Part model, mm, in its own coordinate system. Coordinates: 2 decimals unless noted, no trailing zeros. Order: outer loops, then holes, each group sorted by start corner. A loop starts at its lowest first (then second) coordinate and runs counter-clockwise, first axis right, second up.
from build123d import *

# Parameters (mm, degrees)
BOSS_EXTRUDE1_DEPTH = 129
FILLET1_R           = 0.2
FILLET1_R_2         = 0.3
FILLET1_R_3         = 1
FILLET1_R_4         = 0.5
CHAMFER1_SIZE       = 0.8
CHAMFER1_SIZE2      = 0.601769912


with BuildPart() as part:
    # Sketch1 → Boss-Extrude1 (new body)
    with BuildSketch(Plane.XY):
        Polygon((1.5, 20.5), (1.5, 5.5), (2.375, 5.5), (4.125, 2.75), (5.875, 5.5), (8.5, 5.5), (8.5, 20.5), (9.25, 20.5), (10, 17.8), (10, 0), (8.5, 0), (6.75, 4), (3.25, 0), (1.5, 4), (0, 4), (0, 17.8), (0.75, 20.5), align=None)
    extrude(amount=BOSS_EXTRUDE1_DEPTH)

    # Fillet1
    # the kernel refuses this fillet: 1, 0.5, 0.3, 0.2 mm, written as the material it adds along each edge
    with BuildSketch(Plane(origin=(6.75, 4, 0), x_dir=(0.40081883401970875, -0.9161573349021888, 0), z_dir=(0, 0, 1))) as fillet1_piece_1:
        with BuildLine():
            CenterArc((FILLET1_R * 1.57528283018, -FILLET1_R), FILLET1_R, 90, 115.184697104)
            Line((FILLET1_R * 0.670342090327, -FILLET1_R * 1.42553760981), (0, 0))
            Line((0, 0), (FILLET1_R * 1.57528283018, 0))
        make_face()
    extrude(amount=129)
    # the kernel refuses this fillet: 1, 0.5, 0.3, 0.2 mm, written as the material it takes off along each edge
    with BuildSketch(Plane(origin=(3.25, 0, -1.181462123), x_dir=(0.6585046078685179, 0.752576694706878, 0), z_dir=(0, 0, 1))) as fillet1_2_piece_1:
        with BuildLine():
            CenterArc((FILLET1_R_2 * 1.57528283018, FILLET1_R_2), FILLET1_R_2, 154.815302896, 115.184697104)
            Line((FILLET1_R_2 * 0.670342090327, FILLET1_R_2 * 1.42553760981), (0, 0))
            Line((0, 0), (FILLET1_R_2 * 1.57528283018, 0))
        make_face()
    extrude(amount=131.362924245, mode=Mode.SUBTRACT)
    with BuildSketch(Plane(origin=(8.5, 0, -1.635038937), x_dir=(1, 0, 0), z_dir=(0, 0, 1))) as fillet1_2_piece_2:
        with BuildLine():
            CenterArc((FILLET1_R_3 * 0.654015574786, FILLET1_R_3), FILLET1_R_3, 203.629377731, 66.370622269)
            Line((-FILLET1_R_3 * 0.262141760116, FILLET1_R_3 * 0.59918116598), (0, 0))
            Line((0, 0), (FILLET1_R_3 * 0.654015574786, 0))
        make_face()
    extrude(amount=132.270077874, mode=Mode.SUBTRACT)
    with BuildSketch(Plane(origin=(10, 0, -2.5), x_dir=(0, 1, 0), z_dir=(0, 0, 1))) as fillet1_2_piece_3:
        with BuildLine():
            CenterArc((FILLET1_R_3, FILLET1_R_3), FILLET1_R_3, 180, 90)
            Line((0, FILLET1_R_3), (0, 0))
            Line((0, 0), (FILLET1_R_3, 0))
        make_face()
    extrude(amount=134, mode=Mode.SUBTRACT)
    with BuildSketch(Plane(origin=(0, 4, -1.25), x_dir=(1, 0, 0), z_dir=(0, 0, 1))) as fillet1_2_piece_4:
        with BuildLine():
            CenterArc((FILLET1_R_4, FILLET1_R_4), FILLET1_R_4, 180, 90)
            Line((0, FILLET1_R_4), (0, 0))
            Line((0, 0), (FILLET1_R_4, 0))
        make_face()
    extrude(amount=131.5, mode=Mode.SUBTRACT)
    with BuildSketch(Plane(origin=(9.25, 20.5, -0.380042825), x_dir=(-1, 0, 0), z_dir=(0, 0, 1))) as fillet1_2_piece_5:
        with BuildLine():
            CenterArc((FILLET1_R * 0.760085649571, FILLET1_R), FILLET1_R, 195.524110997, 74.475889003)
            Line((-FILLET1_R * 0.203432260059, FILLET1_R * 0.732356136214), (0, 0))
            Line((0, 0), (FILLET1_R * 0.760085649571, 0))
        make_face()
    extrude(amount=129.76008565, mode=Mode.SUBTRACT)
    with BuildSketch(Plane(origin=(8.5, 20.5, -0.5), x_dir=(0, -1, 0), z_dir=(0, 0, 1))) as fillet1_2_piece_6:
        with BuildLine():
            CenterArc((FILLET1_R, FILLET1_R), FILLET1_R, 180, 90)
            Line((0, FILLET1_R), (0, 0))
            Line((0, 0), (FILLET1_R, 0))
        make_face()
    extrude(amount=130, mode=Mode.SUBTRACT)
    with BuildSketch(Plane(origin=(1.5, 20.5, -0.5), x_dir=(0, -1, 0), z_dir=(0, 0, 1))) as fillet1_2_piece_7:
        with BuildLine():
            CenterArc((FILLET1_R, -FILLET1_R), FILLET1_R, 90, 90)
            Line((0, -FILLET1_R), (0, 0))
            Line((0, 0), (FILLET1_R, 0))
        make_face()
    extrude(amount=130, mode=Mode.SUBTRACT)
    with BuildSketch(Plane(origin=(0.75, 20.5, -0.380042825), x_dir=(1, 0, 0), z_dir=(0, 0, 1))) as fillet1_2_piece_8:
        with BuildLine():
            CenterArc((FILLET1_R * 0.760085649571, -FILLET1_R), FILLET1_R, 90, 74.475889003)
            Line((-FILLET1_R * 0.203432260059, -FILLET1_R * 0.732356136214), (0, 0))
            Line((0, 0), (FILLET1_R * 0.760085649571, 0))
        make_face()
    extrude(amount=129.76008565, mode=Mode.SUBTRACT)

    # Chamfer1
    chamfer1_edges = [part.edges().sort_by_distance(p)[0] for p in [
        (4.125, 2.75, 64.5),
    ]]
    chamfer1_side = [part.faces().sort_by_distance(p)[0] for p in [
        (5, 4.125, 64.5),
    ]]
    chamfer(chamfer1_edges, length=CHAMFER1_SIZE, length2=CHAMFER1_SIZE2, reference=chamfer1_side[0])


solid = part.part
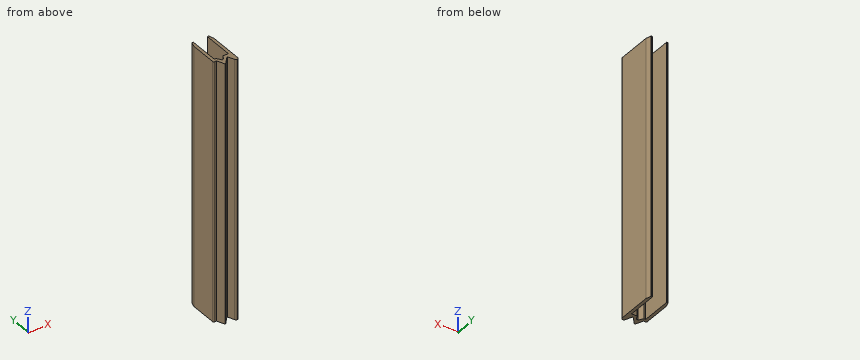
Q1. Cut at A-A on y = 9.5. Write the cut outline in (x, z).
Results list:
outline: (0, 0) - (1.5, 0) - (1.5, 129) - (0, 129) - close; (8.5, 0) - (10, 0) - (10, 129) - (8.5, 129) - close
Q2. Wall check: line 1 along X through (y, z) = (15, 112); line 2 along Y through (x, z) = (1.25, 67); line 3 along X through (y, z) = (1.5, 64). Give the ranges that are in metal, low to high.
Results list:
line 1: x = 0 to 1.5, 8.5 to 10
line 2: y = 4 to 20.5
line 3: x = 2.59 to 4.56, 7.84 to 10
Q3. Pin check, flat tips, straight feed: pin 1 Ø0.7 at (x, z) = (2, 90) entering from +Y; pin 2 Ø0.5 at (x, z) = (1, 56.5) entering from -Y; pin 3 Ø1.5 at (x, z) = (5, 107) entering from -Y. Stop position of each tip, or through.
Results list:
pin 1: stops at y = 5.5
pin 2: stops at y = 4
pin 3: stops at y = 1.14
